Could you check a few things on this model? Use its own coordinates, in mm. Round coordinates to 2 decimals unless told otherwise and drop trailing zeros. Order: outer loops, then holes, each group sorted by start corner. A loop starts at its lowest first (then second) coordinate and runs counter-clockwise, first axis right, second up. Notation, with made-up numbers: M 28.5,67.5 L 84.5,67.5 A33 ccw 84.5,102.5 Z; hole C 67,72.25 d6. An arc over 180 degrees is marked long. Write each question's results on one line, items separated by ' | '. Start each with the question number.
1. I'm going to push flat-ended pins straight in: pin 1 (3 mm diameter, centred on x = 10, z = -2.5, fed in from -Y); pin 2 (1.5 mm diameter, centred on x = -7, y = 0.5, fed in from +Z); pin 3 (1.5 mm diameter, centred on x = 10.5, y = 2.5, fed in from +Z). Where does each tip first touch, or does it pass through?
2. Suppose I cut it at A-A on z = 0. Write out the boundary of the cut face in (x, y) (1 decimal), and give its area (3 significant figures).
3. Suppose I cut it at B-B on x = 0. Write out the boundary of the cut face in (y, z) (1 decimal).
4. Please list where these lines run through material, in increasing order: L1, parallel to X at y = 2.05, z = 0 (3 decimals); L2, parallel to Z at x = 1, y = 2.75; L3, parallel to Z at x = 11, y = 1.55.
5. Suppose I cut it at C-C on y = 2.6. Write out the boundary of the cut face in (x, z) (3 decimals).
6. We'd pull the mould along Z, two halves only. Please class faces 1 (the cylindrical face through (-15, 2.4, 16.4)), 2 (the cylindrical face through (-10.859, 1.565, 1.173)), 3 (the flat face through (5, 3.175, 0)): released by +Z, released by -Z, zero draft, split by the parting line, or undercut.
from build123d import *

# Parameters (mm, degrees)
CUT_EXTRUDE1_DEPTH      = 32.590851198
CUT_EXTRUDE1_DEPTH_BACK = 32.590851198
SKETCH2_R               = 2.1828125


with BuildPart() as part:
    # Sketch1 → Revolve1 (revolve)
    with BuildSketch(Plane.XY, mode=Mode.PRIVATE) as revolve1_sk:
        with BuildLine():
            Line((0, 0), (20.6375, 0))
            ThreePointArc((20.6375, 0), (21.760032015, 0.464967985), (22.225, 1.5875))
            Line((22.225, 1.5875), (22.225, 3.175))
            Line((22.225, 3.175), (0, 3.175))
            Line((0, 3.175), (0, 0))
        make_face()
    revolve(revolve1_sk.sketch.rotate(Axis((0, 0, 0), (0, 1, 0)), 90), axis=Axis((0, 0, 0), (0, 1, 0)))

    # Sketch2 → Cut-Extrude1 (cut, two sides: drawn at the far end of the back side and taken through both)
    with BuildSketch(Plane(origin=(0, 3.175, 0), x_dir=(1, 0, 0), z_dir=(0, 1, 0)).offset(-CUT_EXTRUDE1_DEPTH_BACK)):
        with Locations(Location((0, 0, 0), (0, 0, 270))):
            Circle(SKETCH2_R)
        with Locations(Location((12.7, 0, 0), (0, 0, 270))):
            Circle(SKETCH2_R)
        with Locations(Location((-12.7, 0, 0), (0, 0, 270))):
            Circle(SKETCH2_R)
        with Locations(Location((0, 12.7, 0), (0, 0, 270))):
            Circle(SKETCH2_R)
        with Locations(Location((0, -12.7, 0), (0, 0, 270))):
            Circle(SKETCH2_R)
    extrude(amount=CUT_EXTRUDE1_DEPTH + CUT_EXTRUDE1_DEPTH_BACK, mode=Mode.SUBTRACT)


solid = part.part
Filled sheet:
1) pin 1: stops at y = 0 | pin 2: stops at z = 21.16 | pin 3: stops at z = 19.97
2) outline: M -22.2,1.6 A1.6 ccw -20.6,0 L -14.9,0 L -14.9,3.2 L -22.2,3.2 Z; M -10.5,0 L -2.2,0 L -2.2,3.2 L -10.5,3.2 Z; M 2.2,0 L 10.5,0 L 10.5,3.2 L 2.2,3.2 Z; M 14.9,0 L 20.6,0 A1.6 ccw 22.2,1.6 L 22.2,3.2 L 14.9,3.2 Z | area: 98.5 mm^2
3) outline: M 0,-20.6 A1.6 ccw 1.6,-22.2 L 3.2,-22.2 L 3.2,-14.9 L 0,-14.9 Z; M 0,-10.5 L 3.2,-10.5 L 3.2,-2.2 L 0,-2.2 Z; M 0,2.2 L 3.2,2.2 L 3.2,10.5 L 0,10.5 Z; M 0,14.9 L 3.2,14.9 L 3.2,22.2 L 1.6,22.2 A1.6 ccw 0,20.6 Z
4) L1: x = -22.225 to -14.883, -10.517 to -2.183, 2.183 to 10.517, 14.883 to 22.225 | L2: z = -22.2 to -14.64, -10.76 to -1.94, 1.94 to 10.76, 14.64 to 22.2 | L3: z = -19.31 to -1.37, 1.37 to 19.31
5) outline: C 0,0 d44.45; hole C -12.7,0 d4.366; hole C 0,-12.7 d4.366; hole C 0,0 d4.366; hole C 0,12.7 d4.366; hole C 12.7,0 d4.366
6) face 1: split by the parting line | face 2: undercut | face 3: zero draft
